Verification items for the finished model (mm, model axes). Face numbers are marked on the shaded views. A direction names the side the tool comes from. Coordinates: 2 decimals unless noted, no trailing zeros. Write each loop counter-clockwise with the first axis right and the second up, starting at its lowest first coordinate (ties: lowest second). Pieces come first, ordered by that corner, then holes. Notation, with made-up numbers: (-4, -25.5) - (21, -25.5) arc R12 ccw to (21, -21.5) - close; hole circle Ø8 at (5, 79). An arc over 180 degrees is marked (long way). Use CSV: the item, a comma, the result in double quotes. Start each with the question number.
```python
from build123d import *

# Parameters (mm, degrees)
F0_W      = 88.9
F0_H      = 50.8
F1_DEPTH  = 25.4
F2_W      = 63.5
F2_H      = 25.4
F3_DEPTH  = 25.401
F4_W      = 88.9
F4_H      = 12.7
F5_DEPTH  = 25.401
F8_W      = 19.05
F8_H      = 11.447972618
F9_DEPTH  = 12.701
F10_W     = 12.7
F10_H     = 11.090603964
F11_DEPTH = 38.101
F12_R     = 3.175
F14_DEPTH = 12.701
F13_R     = 3.175
F15_DEPTH = 12.701


# Not quite as in the source:
# - a feature of the source that left no trace in its solid (it failed there, or was rolled back) is left out


with BuildPart() as f1:
    # F0 (on Front) → F1 (new body)
    with BuildSketch(Plane.XZ):
        Rectangle(F0_W, F0_H)
    extrude(amount=F1_DEPTH)

    # F2 (on face) → F3 (cut, through all)
    with BuildSketch(Plane.XZ.offset(25.4)):
        with Locations((0, 12.7)):
            Rectangle(F2_W, F2_H)
    extrude(amount=-F3_DEPTH, mode=Mode.SUBTRACT)

    # F4 (on face) → F5 (cut, through all)
    with BuildSketch(Plane.XZ.offset(25.4)):
        with Locations((0, -19.05)):
            Rectangle(F4_W, F4_H)
    extrude(amount=-F5_DEPTH, mode=Mode.SUBTRACT)

    # F8 (on face) → F9 (cut, through all)
    with BuildSketch(Plane.XY):
        with Locations((32.2608303964, -19.8649899103)):
            Rectangle(F8_W, F8_H)
    extrude(amount=-F9_DEPTH, mode=Mode.SUBTRACT)

    # F10 (on face) → F11 (cut, through all)
    with BuildSketch(Plane.XY.offset(25.4)):
        with Locations((38.1, -19.854698018)):
            Rectangle(F10_W, F10_H)
    extrude(amount=-F11_DEPTH, mode=Mode.SUBTRACT)

    # F12 (on face) → F14 (cut, through all)
    with BuildSketch(Plane.XY):
        with Locations((24.2214165628, -5.1358360797)):
            Circle(F12_R)
    extrude(amount=-F14_DEPTH, mode=Mode.SUBTRACT)

    # F13 (on face) → F15 (cut, through all)
    with BuildSketch(Plane.XY):
        with Locations((-20.2783960849, -10.4468446225)):
            Circle(F13_R)
    extrude(amount=-F15_DEPTH, mode=Mode.SUBTRACT)


solid = f1.part
```
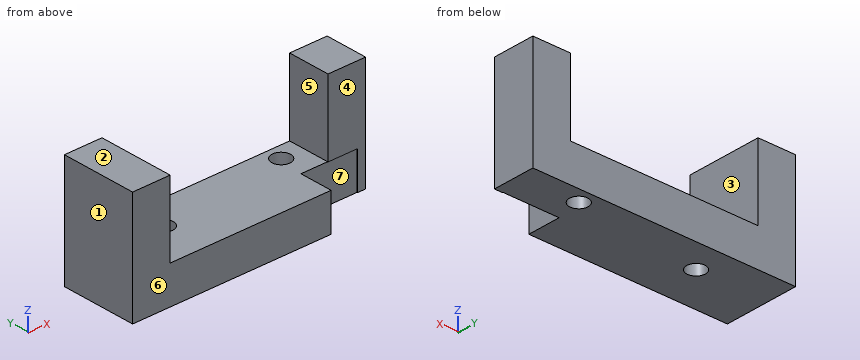
Q1. Tool access check on the marked faces 4, 5, 6 and 7. Record the directions out of +Z, -Z, +X, -X, +Y, -Y that give a thin tool (end or side, any length) a straight path to the whole face; none if there is none.
Q2. Release check for a two-part mould opening along X. For the marked faces 1, 2 and 3 record: released by +X, released by -X, zero draft, split by the parting line, or undercut.
Q3. Scan lines: line 1 along X through (y, z) = (-8.75, 19); line 2 along Z through (x, y) = (31, -14); line 3 along X through (y, z) = (-15, -3.5). Record each from-to range of solid material in increasing order. Write a range as from..to.
Q4. Cross-section at C-C (y = -11.5). Record the cut outline in (x, z), plus the area to 3 significant figures.
Q5. Cross-section at D-D (x = 34). Record the cut outline in (y, z).
Q6. Gauge pin test, flat ends, axial feed: pin 1 (1 mm diameter, centred on y = -17, z = 1.5, fed in from +X); pin 2 (5.5 mm diameter, centred on y = -22.5, z = -4.5, fed in from +X); pin 3 (5.5 mm diameter, centred on x = 24.22, y = -5.14, fed in from -Z); pin 4 (14 mm diameter, centred on x = 39.5, z = 13, fed in from -Y). Record the tip position at first contact, or that the pin passes through.
Q7. Cross-section at A-A (z = 12). Record the cut outline in (x, y), plus the area to 3 significant figures.
Q8. Cross-section at B-B (y = -16.75). Record the cut outline in (x, z), plus the area to 3 significant figures.
Reply:
1,face 4,"+Z, -Z, +X, -Y"
1,face 5,"+Z, +Y, -Y"
1,face 6,"+Z, -Z, +X, -X, -Y"
1,face 7,"-Z, -Y"
2,face 1,"released by -X"
2,face 2,"zero draft"
2,face 3,"undercut"
3,line 1,"-44.45..-31.75, 31.75..44.45"
3,line 2,"-12.7..0"
3,line 3,"-44.45..22.74"
4,outline,"(-44.45, -12.7) - (-23.27, -12.7) - (-23.27, 0) - (-31.75, 0) - (-31.75, 25.4) - (-44.45, 25.4) - close; (-17.28, -12.7) - (44.45, -12.7) - (44.45, 25.4) - (31.75, 25.4) - (31.75, 0) - (-17.28, 0) - close"
4,area,"1,700 mm^2"
5,outline,"(-14.31, 0) - (-14.14, 0) - (-14.14, -12.7) - (0, -12.7) - (0, 25.4) - (-14.31, 25.4) - close"
6,pin 1,"x = -31.75"
6,pin 2,"x = 22.74"
6,pin 3,"through"
6,pin 4,"y = -14.31"
7,outline,"(-44.45, -25.4) - (-31.75, -25.4) - (-31.75, 0) - (-44.45, 0) - close; (31.75, -14.31) - (44.45, -14.31) - (44.45, 0) - (31.75, 0) - close"
7,area,"504 mm^2"
8,outline,"(-44.45, -12.7) - (22.74, -12.7) - (22.74, 0) - (-31.75, 0) - (-31.75, 25.4) - (-44.45, 25.4) - close"
8,area,"1,180 mm^2"
